```python
from build123d import *

# Parameters (mm, degrees)
SCHIZZO1_W                   = 541
SCHIZZO1_H                   = 320
ESTRUSIONE_ESTRUSIONE1_DEPTH = 275
SCHIZZO2_W                   = 35
SCHIZZO2_H                   = 58.8
ESTRUSIONE_ESTRUSIONE2_DEPTH = 28
SCHIZZO3_R                   = 15
ESTRUSIONE_ESTRUSIONE3_DEPTH = 21
SCHIZZO4_R                   = 4
TAGLIO_ESTRUSIONE1_DEPTH     = 15
SCHIZZO5_R                   = 4
TAGLIO_ESTRUSIONE2_DEPTH     = 15


with BuildPart() as part:
    # Schizzo1 → Estrusione-Estrusione1 (new body)
    with BuildSketch(Plane(origin=(0, 0, 0), x_dir=(1, 0, 0), z_dir=(0, 1, 0))):
        Rectangle(SCHIZZO1_W, SCHIZZO1_H)
    extrude(amount=ESTRUSIONE_ESTRUSIONE1_DEPTH)

    # Schizzo2 → Estrusione-Estrusione2 (add)
    with BuildSketch(Plane(origin=(270.5, 0, 0), x_dir=(0, 0, -1), z_dir=(1, 0, 0))):
        with Locations((-73.5, 169.05)):
            Rectangle(SCHIZZO2_W, SCHIZZO2_H)
        with Locations((73.5, 169.05)):
            Rectangle(SCHIZZO2_W, SCHIZZO2_H)
    extrude(amount=ESTRUSIONE_ESTRUSIONE2_DEPTH)

    # Schizzo3 → Estrusione-Estrusione3 (add)
    with BuildSketch(Plane(origin=(270.5, 0, 0), x_dir=(0, 0, -1), z_dir=(1, 0, 0))):
        with Locations(Location((0, 180, 0), (0, 0, 180))):
            Circle(SCHIZZO3_R)
        Polygon((0, 147.320508076), (-15, 138.660254038), (-15, 121.339745962), (0, 112.679491924), (15, 121.339745962), (15, 138.660254038), align=None)
    extrude(amount=ESTRUSIONE_ESTRUSIONE3_DEPTH)

    # Schizzo4 → Taglio-Estrusione1 (cut)
    with BuildSketch(Plane(origin=(270.5, 0, 0), x_dir=(0, 0, -1), z_dir=(1, 0, 0))):
        with Locations((-145, 15)):
            Circle(SCHIZZO4_R)
        with Locations((145, 15)):
            Circle(SCHIZZO4_R)
    taglio_estrusione1 = extrude(amount=-TAGLIO_ESTRUSIONE1_DEPTH, mode=Mode.SUBTRACT)

    # Specchia1: Taglio-Estrusione1 across plane
    add(taglio_estrusione1.mirror(Plane(origin=(0, 0, 0), x_dir=(0, 0, 1), z_dir=(1, 0, 0))), mode=Mode.SUBTRACT)

    # Schizzo5 → Taglio-Estrusione2 (cut)
    with BuildSketch(Plane.XY.offset(160)):
        with Locations((-240.5, 15)):
            Circle(SCHIZZO5_R)
        with Locations((240.5, 15)):
            Circle(SCHIZZO5_R)
    extrude(amount=-TAGLIO_ESTRUSIONE2_DEPTH, mode=Mode.SUBTRACT)


solid = part.part
```
Geometry check sheet. Reference: the model listing, model coordinates, mm. A direction names the side the tool comes from. Give positions to 0.01 mm unless a question says otherwise; leave off trailing zeros. Loops run counter-clockwise (first coordinate to the right, second up) from the corner with the lowest first, then second, coordinate; pieces in that order, holes last. Notation, with made-up numbers: M 77,-0.5 L 133,-0.5 A26 ccw 133,32.5 Z; hole C 53.25,49 d4. An arc over 180 degrees is marked long. Write item = value, one per line. Start each with the question number.
1. Section check B-B, the plane z = -131. Enter the section's corners in (x, y), plus the area to 3 significant figures.
2. Thickness scan on probe 1 along Y at (x, z) = (262, -145); probe 2 along X at (y, z) = (118, -72.5). Record the ranges inside material, lowest first.
3. Section check C-C, the plane y = 61.5. Enter the section's corners in (x, z).
4. Tool access check on faces 1 (the face through (291.5, 180, 0)), 2 (the face through (281, 130, 15)), 3 (the face through (280.853, 142.93, -7.605)). Record the directions out of +Z, -Z, +X, -X, +Y, -Y that give a thin tool (end or side, any length) a straight path to the whole face; none if there is none.
5. Section check A-A, the plane y = 180. Enter the section's corners in (x, z).
6. Go/stop test with flat-tipped pins: P1, Ø6.5, axis at y = 13.5, z = -146, coming from the +X side; P2, Ø8.5, axis at x = 289.5, y = 170.5, coming from the -Z side; P3, Ø22.5, axis at x = 281, z = -76, coming from the +Y side; P4, Ø4, axis at y = 16.5, z = 146, coming from the +X side. Record where each tip stops, or that it passes through.
Values follow:
q1.outline = M -270.5,0 L 270.5,0 L 270.5,275 L -270.5,275 Z
q1.area = 149,000 mm^2
q2.probe_1 = 0 to 11, 19 to 275
q2.probe_2 = -270.5 to 270.5
q3.outline = M -270.5,-160 L 270.5,-160 L 270.5,160 L -270.5,160 Z
q4.face_1 = +X, +Y, -Y
q4.face_2 = +Z, +X, +Y, -Y
q4.face_3 = +X
q5.outline = M -270.5,-160 L 270.5,-160 L 270.5,-91 L 298.5,-91 L 298.5,-56 L 270.5,-56 L 270.5,-15 L 291.5,-15 L 291.5,15 L 270.5,15 L 270.5,56 L 298.5,56 L 298.5,91 L 270.5,91 L 270.5,160 L -270.5,160 Z
q6.P1 = 270.5
q6.P2 = -91
q6.P3 = 275
q6.P4 = 255.5
